```python
from build123d import *

# Parameters (mm, degrees)
BOSS_EXTRUDE1_DEPTH      = 95
BOSS_EXTRUDE2_DEPTH      = 32
SKETCH3_W                = 10
SKETCH3_H                = 16
SKETCH3_H_2              = 32
CUT_EXTRUDE1_DEPTH       = 4
CUT_EXTRUDE2_DEPTH       = 28
BOSS_EXTRUDE3_DEPTH      = 2
BOSS_EXTRUDE3_DEPTH_BACK = 4
SKETCH5_W                = 70
SKETCH5_H                = 16
SKETCH6_R                = 1.75
CUT_EXTRUDE3_DEPTH       = 111.792599031
SKETCH7_R                = 1.75
CUT_EXTRUDE4_DEPTH       = 118.58418261
CUT_EXTRUDE5_DEPTH       = 117.517981445
CUT_EXTRUDE5_DEPTH_BACK  = 117.517981445
FILLET1_R                = 2


with BuildPart() as part:
    # Sketch1 → Boss-Extrude1 (new body)
    with BuildSketch(Plane(origin=(0, 0, 0), x_dir=(0, 1, 0), z_dir=(0, 0, 1))):
        with BuildLine():
            Line((16.8, -16.8), (16.8, 16.8))
            Line((16.8, 16.8), (4, 16.8))
            Line((4, 16.8), (4, 26.8))
            Line((4, 26.8), (0, 26.8))
            Line((0, 26.8), (0, 12.8))
            ThreePointArc((0, 12.8), (12.8, 0), (0, -12.8))
            Line((0, -12.8), (0, -26.8))
            Line((0, -26.8), (4, -26.8))
            Line((4, -26.8), (4, -16.8))
            Line((4, -16.8), (16.8, -16.8))
        make_face()
    extrude(amount=BOSS_EXTRUDE1_DEPTH)

    # Sketch2 → Boss-Extrude2 (add)
    with BuildSketch(Plane(origin=(0, 0, 0), x_dir=(1, 0, 0), z_dir=(0, 0, -1))):
        with BuildLine():
            Line((-16.8, -16.8), (-16.8, -22.660571771))
            ThreePointArc((-16.8, -22.660571771), (0, -63.8), (16.8, -22.660571771))
            Line((16.8, -22.660571771), (16.8, -16.8))
            Line((16.8, -16.8), (-16.8, -16.8))
        make_face()
    extrude(amount=-BOSS_EXTRUDE2_DEPTH)

    # Sketch3 → Cut-Extrude1 (cut)
    with BuildSketch(Plane.XZ):
        with Locations((-21.8, 87)):
            Rectangle(SKETCH3_W, SKETCH3_H)
        with Locations((-21.8, 16)):
            Rectangle(SKETCH3_W, SKETCH3_H_2)
        with Locations((21.8, 16)):
            Rectangle(SKETCH3_W, SKETCH3_H_2)
        with Locations((21.8, 87)):
            Rectangle(SKETCH3_W, SKETCH3_H)
    extrude(amount=-CUT_EXTRUDE1_DEPTH, mode=Mode.SUBTRACT)

    # Sketch4 → Cut-Extrude2 (cut)
    with BuildSketch(Plane.XY.offset(32)):
        Polygon((-11.38, 54.574393389), (-18.485, 42.268172401), (-18.485, 37.331827599), (-11.38, 25.025606611), (-7.105, 22.557434211), (7.105, 22.557434211), (11.38, 25.025606611), (18.485, 37.331827599), (18.485, 42.268172401), (11.38, 54.574393389), (7.105, 57.042565789), (-7.105, 57.042565789), align=None)
    extrude(amount=-CUT_EXTRUDE2_DEPTH, mode=Mode.SUBTRACT)

    # Sketch5 → Boss-Extrude3 (add, two sides: drawn at the far end of the back side and taken through both)
    with BuildSketch(Plane(origin=(0, 16.8, 0), x_dir=(-1, 0, 0), z_dir=(0, 1, 0)).offset(-BOSS_EXTRUDE3_DEPTH_BACK)):
        with Locations((0, 87)):
            Rectangle(SKETCH5_W, SKETCH5_H)
    extrude(amount=BOSS_EXTRUDE3_DEPTH + BOSS_EXTRUDE3_DEPTH_BACK)

    # Sketch6 → Cut-Extrude3 (cut, through all)
    with BuildSketch(Plane(origin=(0, 18.8, 0), x_dir=(-1, 0, 0), z_dir=(0, 1, 0))):
        with Locations(Location((-30, 87, 0), (0, 0, 90))):
            Circle(SKETCH6_R)
        with Locations(Location((30, 87, 0), (0, 0, 90))):
            Circle(SKETCH6_R)
    extrude(amount=-CUT_EXTRUDE3_DEPTH, mode=Mode.SUBTRACT)

    # Sketch7 → Cut-Extrude4 (cut, through all)
    with BuildSketch(Plane(origin=(0, 4, 0), x_dir=(-1, 0, 0), z_dir=(0, 1, 0))):
        with Locations(Location((-21.8, 72, 0), (0, 0, 90))):
            Circle(SKETCH7_R)
        with Locations(Location((-21.8, 39, 0), (0, 0, 90))):
            Circle(SKETCH7_R)
        with Locations(Location((21.8, 39, 0), (0, 0, 270))):
            Circle(SKETCH7_R)
        with Locations(Location((21.8, 72, 0), (0, 0, 270))):
            Circle(SKETCH7_R)
    extrude(amount=-CUT_EXTRUDE4_DEPTH, mode=Mode.SUBTRACT)

    # Sketch8 → Cut-Extrude5 (cut, two sides: drawn at the far end of the back side and taken through both)
    with BuildSketch(Plane.XY.offset(4).offset(-CUT_EXTRUDE5_DEPTH_BACK)):
        with BuildLine():
            Line((-4, 35.8), (4, 35.8))
            Line((4, 35.8), (4, 63.464319132))
            ThreePointArc((4, 63.464319132), (0, 63.8), (-4, 63.464319132))
            Line((-4, 63.464319132), (-4, 35.8))
        make_face()
    extrude(amount=CUT_EXTRUDE5_DEPTH + CUT_EXTRUDE5_DEPTH_BACK, mode=Mode.SUBTRACT)

    # Fillet1
    fillet1_edges = [part.edges().sort_by_distance(p)[0] for p in [
        (-9.2425, 55.808479589, 32),
        (-14.9325, 48.421282895, 32),
        (-18.485, 39.8, 32),
        (-14.9325, 31.178717105, 32),
        (-9.2425, 23.791520411, 32),
        (0, 22.557434211, 32),
        (9.2425, 23.791520411, 32),
        (14.9325, 31.178717105, 32),
        (18.485, 39.8, 32),
        (14.9325, 48.421282895, 32),
        (9.2425, 55.808479589, 32),
        (5.5525, 57.042565789, 32),
        (-5.5525, 57.042565789, 32),
        (-4, 63.464319132, 16),
        (4, 63.464319132, 16),
    ]]
    fillet(fillet1_edges, radius=FILLET1_R)


solid = part.part
```
Work out the finished part from the listing and answer in its coordinate system (mm). A direction names the side the tool comes from. Give positions to 0.01 mm unless a question says otherwise; leave off trailing zeros. Write each loop counter-clockwise with the first axis right and the second up, starting at its lowest first coordinate (ties: lowest second). Pieces come first, ordered by that corner, then holes. Notation, with made-up numbers: (-38, -5) -> (16, -5) arc R8 ccw to (16, 6) -> close; hole circle Ø4 at (13.25, 73). An arc over 180 degrees is marked (long way). Write each question's results on one line, items separated by ' | '.
1. Find section A-A on z = 39. Determine the outline of the cut face in (x, y).
Data:
outline: (-26.8, 0) -> (-23.55, 0) -> (-23.55, 4) -> (-26.8, 4) -> close; (-20.05, 0) -> (-12.8, 0) arc R12.8 cw to (12.8, 0) -> (20.05, 0) -> (20.05, 4) -> (16.8, 4) -> (16.8, 16.8) -> (-16.8, 16.8) -> (-16.8, 4) -> (-20.05, 4) -> close; (23.55, 0) -> (26.8, 0) -> (26.8, 4) -> (23.55, 4) -> close
2. Find section C-C on z = 87. Determine the outline of the cut face in (x, y), and give its area (3 significant figures).
Data:
outline: (-35, 12.8) -> (-31.75, 12.8) -> (-31.75, 18.8) -> (-35, 18.8) -> close; (-28.25, 12.8) -> (-16.8, 12.8) -> (-16.8, 0) -> (-12.8, 0) arc R12.8 cw to (12.8, 0) -> (16.8, 0) -> (16.8, 12.8) -> (28.25, 12.8) -> (28.25, 18.8) -> (-28.25, 18.8) -> close; (31.75, 12.8) -> (35, 12.8) -> (35, 18.8) -> (31.75, 18.8) -> close | area: 551 mm^2
3. Each of these flat-tipped pins is pushed along its axis until it touches: pin 1 Ø1 at (x, y) = (-6.5, 23.5) entering from +Z; pin 2 Ø5.5 at (x, z) = (30, 87) entering from +Y; pin 3 Ø1.2 at (x, y) = (19.5, 1) entering from -Z; pin 4 Ø3 at (x, z) = (-21.8, 72) entering from -Y. Where does it stop, or does it pass through?
Data:
pin 1: z = 4 | pin 2: y = 18.8 | pin 3: z = 32 | pin 4: through
4. Determine the mould class of faces 1 (the flat face through (6, 57.043, 17)), 2 (the flat face through (-22, 2, 79)), 3 (the flat face through (0, 31, 0)) for opening direction Z: +Z half, -Z half, draft (parallel to the pull), parting line (faces both ways), or undercut.
Data:
face 1: draft | face 2: +Z half | face 3: -Z half
5. Straight lines are drawn through the part: L1, parallel to X at y = 15.9, z = 87; L2, parallel to X at y = 2.4, z = 39; L3, parallel to Z at x = 21, y = 2. For each, find the intervals that lie inside material, in ascending order.
Data:
L1: -35 to -31.75, -28.25 to 28.25, 31.75 to 35 | L2: -26.8 to -23.55, -20.05 to -12.57, 12.57 to 20.05, 23.55 to 26.8 | L3: 32 to 37.44, 40.56 to 70.44, 73.56 to 79
6. Find section B-B on x = 30. Determine the outline of the cut face in (y, z).
Data:
outline: (12.8, 79) -> (18.8, 79) -> (18.8, 85.25) -> (12.8, 85.25) -> close; (12.8, 88.75) -> (18.8, 88.75) -> (18.8, 95) -> (12.8, 95) -> close
7. Find section D-D on x = 21.8. Determine the outline of the cut face in (y, z).
Data:
outline: (0, 32) -> (4, 32) -> (4, 37.25) -> (0, 37.25) -> close; (0, 40.75) -> (4, 40.75) -> (4, 70.25) -> (0, 70.25) -> close; (0, 73.75) -> (4, 73.75) -> (4, 79) -> (0, 79) -> close; (12.8, 79) -> (18.8, 79) -> (18.8, 95) -> (12.8, 95) -> close; (29.76, 0) -> (49.84, 0) -> (49.84, 32) -> (29.76, 32) -> close
8. A tool of negligible diameter and unlimited length cuts with its end or side. For faces 4 (the flat face through (22, 4, 55)), 5 (the flat face through (22, 2, 79)), 6 (the cylindrical face through (15.51, 30.97, 31.43)), from which of +Z, -Z, +X, -X, +Y, -Y can it reach the whole face along a straight path? Write none if from no direction.
Data:
face 4: +Z, -Z, +X, +Y | face 5: +Z, +X, -Y | face 6: +Z
